```python
from build123d import *

# Parameters (mm, degrees)
SKETCH1_W             = 45
SKETCH1_H             = 30
SKETCH1_R             = 1.525
BOSS_EXTRUDE1_DEPTH   = 3
SKETCH2_R             = 4
BOSS_EXTRUDE2_DEPTH   = 5
SKETCH3_R             = 5
BOSS_EXTRUDE3_DEPTH   = 0.5
F_2_CLEARANCE_HOLE1_D = 2.2606
SKETCH6_R             = 2.5
SKETCH6_R_2           = 1.525
BOSS_EXTRUDE4_DEPTH   = 1


with BuildPart() as part:
    # Sketch1 → Boss-Extrude1 (new body)
    with BuildSketch(Plane.XY):
        with Locations((7.5, 0)):
            Rectangle(SKETCH1_W, SKETCH1_H)
        with Locations((18.050000068, 0)):
            Circle(SKETCH1_R, mode=Mode.SUBTRACT)
    extrude(amount=BOSS_EXTRUDE1_DEPTH)

    # Sketch2 → Boss-Extrude2 (add)
    with BuildSketch(Plane.XY.offset(3)):
        Circle(SKETCH2_R)
    extrude(amount=BOSS_EXTRUDE2_DEPTH)

    # Sketch3 → Boss-Extrude3 (add)
    with BuildSketch(Plane.XY.offset(3)):
        Circle(SKETCH3_R)
    extrude(amount=BOSS_EXTRUDE3_DEPTH)

    # #2 Clearance Hole1 (through all)
    with Locations(Plane.XY.offset(3)):
        with Locations((-12.5, 12.5), (-12.5, -12.5), (27.5, -12.5), (27.5, 12.5)):
            Hole(F_2_CLEARANCE_HOLE1_D / 2)

    # Sketch6 → Boss-Extrude4 (add)
    with BuildSketch(Plane.XY.offset(3)):
        with Locations((18.050000068, 0)):
            Circle(SKETCH6_R)
        with Locations((18.050000068, 0)):
            Circle(SKETCH6_R_2, mode=Mode.SUBTRACT)
    extrude(amount=BOSS_EXTRUDE4_DEPTH)


solid = part.part
```
Source: CAD feature listing. Evaluate the final solid. Frame: model axes, mm. A direction names the side the tool comes from. Coordinates: 2 decimals unless noted, no trailing zeros. Loops run counter-clockwise (first coordinate to the right, second up) from the corner with the lowest first, then second, coordinate; pieces in that order, holes last. Notation, with made-up numbers: M 29,70.25 L 85,70.25 A18 cw 85,82.25 Z; hole C -11.5,9 d11. An arc over 180 degrees is marked long. Put each result on its own line as item: value. Start each with the question number.
1) Ray query, L1, parallel to Y at x = -12.5, z = 1.65; L2, parallel to X at y = -13.5, z = 0.5; L3, parallel to Z at x = 14, y = 2.5. Return the intervals inside material, ascending. Write a range as from..to.
2) Cut plane C-C on y = 0. Return the cut outline in (x, z) (3 decimals), then the cut area to 3 significant figures.
3) Contact query for flat-ended pins moving along their axis: pin 1 Ø5 at (x, y) = (20, -6.5) entering from +Z; pin 2 Ø4 at (x, y) = (17.5, -1) entering from +Z. Output: stop coordinate, or through.
4) Cut plane A-A on y = 12.5. Return the cut outline in (x, z).
5) Reachability of faces 1 (the face through (-1.08, -4.88, 3.25)), 2 (the face through (20, 0, 4)), 3 (the face through (16.526, 0.067, 1.972)) from +Z, -Z, +X, -X, +Y, -Y: full face, straight path, thin tool, end or side. Return the list, or none.
6) Cut plane D-D on x = 0. Return the cut outline in (y, z).
7) Pull-direction query (X, two-part tool) for faces 4 (the face through (7, -15, 1)), 5 (the face through (28.63, 12.55, 1.48)), 6 (the face through (-15, 0, 1)); classes: pulls with the +X half, pulls with the -X half, needs draft (parallel to the pull), parting line crosses it, or undercut.
8) Cut plane B-B on z = 2. Return the cut outline in (x, y) (3 decimals).
The answers:
1. L1: y = -15..-13.63, -11.37..11.37, 13.63..15
1. L2: x = -15..-13.03, -11.97..26.97, 28.03..30
1. L3: z = 0..3
2. outline: M -15,0 L 16.525,0 L 16.525,4 L 15.55,4 L 15.55,3 L 5,3 L 5,3.5 L 4,3.5 L 4,8 L -4,8 L -4,3.5 L -5,3.5 L -5,3 L -15,3 Z; M 19.575,0 L 30,0 L 30,3 L 20.55,3 L 20.55,4 L 19.575,4 Z
2. area: 169 mm²
3. pin 1: stops at z = 3
3. pin 2: stops at z = 4
4. outline: M -15,0 L -13.63,0 L -13.63,3 L -15,3 Z; M -11.37,0 L 26.37,0 L 26.37,3 L -11.37,3 Z; M 28.63,0 L 30,0 L 30,3 L 28.63,3 Z
5. face 1: +Z
5. face 2: +Z, +X, +Y, -Y
5. face 3: +Z, -Z
6. outline: M -15,0 L 15,0 L 15,3 L 5,3 L 5,3.5 L 4,3.5 L 4,8 L -4,8 L -4,3.5 L -5,3.5 L -5,3 L -15,3 Z
7. face 4: needs draft
7. face 5: undercut
7. face 6: pulls with the -X half
8. outline: M -15,-15 L 30,-15 L 30,15 L -15,15 Z; hole C -12.5,-12.5 d2.261; hole C -12.5,12.5 d2.261; hole C 18.05,0 d3.05; hole C 27.5,-12.5 d2.261; hole C 27.5,12.5 d2.261
